The figure shows three views and two pictorial views of one solid part (mm, origin at its lowest corner). Answer the questions. A direction names the side the tool comes from. Coordinates: 2 decimals unless noted, no trailing zeros. Order: outer loops, then holes, each group sorted by start corner. A loop starts at its lowest first (then second) coordinate and runs counter-clockwise, first axis right, second up. Notation, with made-up numbers: M 46.25,63.5 L 72.25,63.5 A21 ccw 72.25,98.5 Z; hole C -31,27.5 d7. An arc over 180 degrees is marked long. Answer in a Markdown table with one row per item. Add a question column.
Item 1: The part is cut by section A-A (z = 0.75). Write down the section's boundary in (x, y), then the cut area to 3 significant figures.
Item 2: Which of the six approach directions +Z, -Z, +X, -X, +Y, -Y give full straight-line access (tool end or side, diameter ignored) to the marked faces 1, 2 and 3?
Item 3: Consider line 1 (X direction, y = 5, z = 0.55); line 2 (X direction, y = 7.5, z = 2.1); line 3 (Y direction, x = 3.5, z = 0.8). Determine where each line is inside the solid, lowest interval first. Write a range as from..to.
Item 4: The part is cut by section C-C (y = 5). Write down the section's boundary in (x, z), then the cut area to 3 significant figures.
Item 5: The part is cut by section D-D (z = 1.5). Write down the section's boundary in (x, y).
Item 6: Flat-ended cylindrical pins translate along their axes: pin 1 Ø2 at (x, y) = (3, 3) entering from +Z; pin 2 Ø2 at (y, z) = (6, 2.5) entering from -X; pin 3 Ø4 at (x, y) = (3, 8) entering from -Z; pin 4 Ø2 at (x, y) = (10, 6.5) entering from -Z. Find the tip coordinate at first contact, or state that the pin passes through.
Item 7: The part is cut by section B-B (x = 3.5). Write down the section's boundary in (y, z).
Item 8: The mould has two halves that part along X. Classify the marked faces 4, 5 and 6: released by +X, released by -X, zero draft, split by the parting line, or undercut.
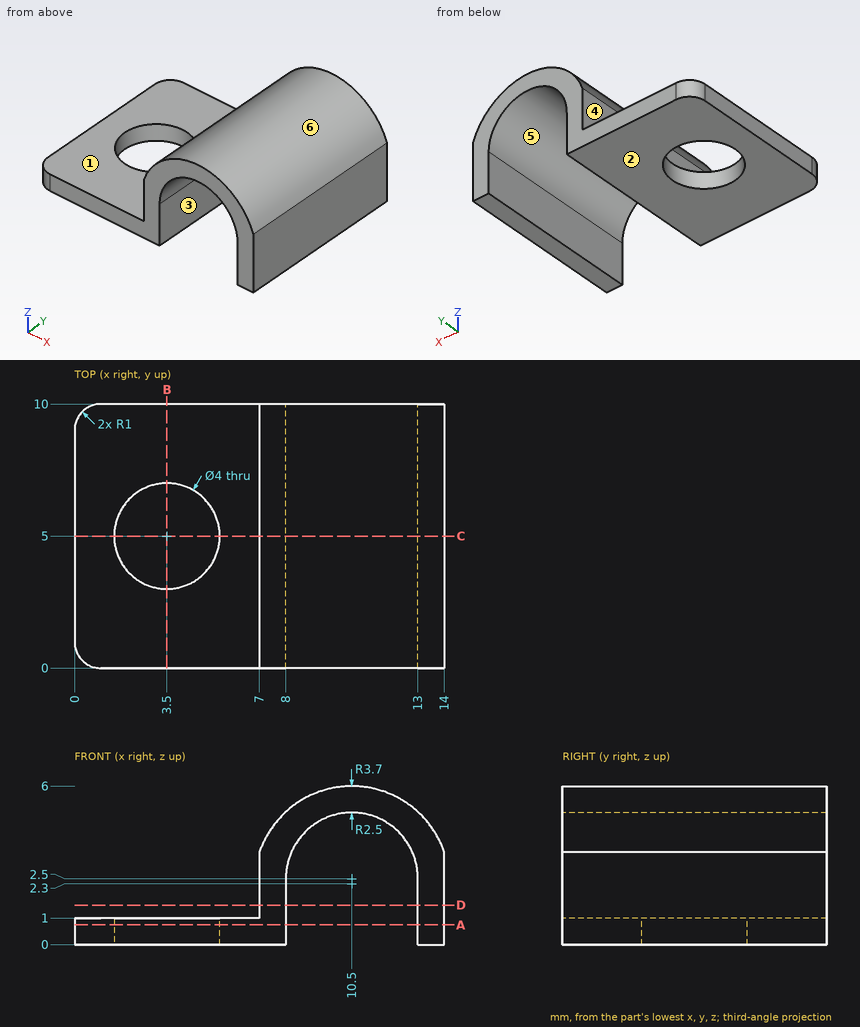
Reply:
| question | item | result |
|---|---|---|
| 1 | outline | M 0,1 A1 ccw 1,0 L 8,0 L 8,10 L 1,10 A1 ccw 0,9 Z; M 13,0 L 14,0 L 14,10 L 13,10 Z; hole C 3.5,5 d4 |
| 1 | area | 77.0 mm2 |
| 2 | face 1 | +Z, -X, +Y, -Y |
| 2 | face 2 | -Z, +X, -X, +Y, -Y |
| 2 | face 3 | -Z, +Y, -Y |
| 3 | line 1 | x = 0..1.5, 5.5..8, 13..14 |
| 3 | line 2 | x = 7..8, 13..14 |
| 3 | line 3 | y = 0..3, 7..10 |
| 4 | outline | M 0,0 L 1.5,0 L 1.5,1 L 0,1 Z; M 5.5,0 L 8,0 L 8,2.5 A2.5 cw 13,2.5 L 13,0 L 14,0 L 14,3.5 A3.7 ccw 7,3.5 L 7,1 L 5.5,1 Z |
| 4 | area | 18.0 mm2 |
| 5 | outline | M 7,0 L 8,0 L 8,10 L 7,10 Z; M 13,0 L 14,0 L 14,10 L 13,10 Z |
| 6 | pin 1 | stops at z = 1 |
| 6 | pin 2 | stops at x = 7 |
| 6 | pin 3 | stops at z = 0 |
| 6 | pin 4 | stops at z = 4.5 |
| 7 | outline | M 0,0 L 3,0 L 3,1 L 0,1 Z; M 7,0 L 10,0 L 10,1 L 7,1 Z |
| 8 | face 4 | released by -X |
| 8 | face 5 | undercut |
| 8 | face 6 | split by the parting line |
